```python
from build123d import *

# Parameters (mm, degrees)
ROW_SKETCH_W            = 16
ROW_SKETCH_H            = 6
ROW_ANGLE               = 59
HEEL_SKETCH_W           = 44
HEEL_SKETCH_H           = 6
HEEL_ANGLE              = 30
LUG_BLOCK_SKETCH_W      = 22
LUG_BLOCK_SKETCH_H      = 33
LUG_BLOCK_DEPTH         = 25
SLOT_SKETCH_W           = 32
SLOT_SKETCH_H           = 33
SLOT_DEPTH              = 20
PIN_HOLE_SKETCH_R       = 3.1
PIN_HOLE_DEPTH          = 30
TAB_SKETCH_W            = 23
TAB_SKETCH_H            = 26
TAB_DEPTH               = 5
SWITCH_HOLES_SKETCH_R   = 1.1
SWITCH_HOLES_DEPTH      = 30
SCREW_HOLE_1_SKETCH_R   = 2.25
SCREW_HOLE_1_DEPTH      = 200
SCREW_HOLE_1_SKETCH_2_R = 2.25
SCREW_HOLE_1_2_DEPTH    = 200


with BuildPart() as part:
    # Row Sketch → Row (revolve, symmetric)
    with BuildSketch(Plane.XY) as row_sk:
        with Locations((-896, 104.7)):
            Rectangle(ROW_SKETCH_W, ROW_SKETCH_H)
    revolve(axis=Axis((-3000, 0, 0), (1, 0, 0)), revolution_arc=ROW_ANGLE / 2)
    revolve(row_sk.sketch, axis=Axis((-3000, 0, 0), (-1, 0, 0)), revolution_arc=ROW_ANGLE / 2)

    # Heel Sketch → Heel (revolve, symmetric)
    with BuildSketch(Plane.XY) as heel_sk:
        with Locations((-866, 104.7)):
            Rectangle(HEEL_SKETCH_W, HEEL_SKETCH_H)
    revolve(axis=Axis((-3000, 0, 0), (1, 0, 0)), revolution_arc=HEEL_ANGLE / 2)
    revolve(heel_sk.sketch, axis=Axis((-3000, 0, 0), (-1, 0, 0)), revolution_arc=HEEL_ANGLE / 2)

    # Lug Block Sketch → Lug Block (add, symmetric)
    with BuildSketch(Plane.XY):
        with Locations((-856, 119.5)):
            Rectangle(LUG_BLOCK_SKETCH_W, LUG_BLOCK_SKETCH_H)
    extrude(amount=LUG_BLOCK_DEPTH, both=True)

    # Slot Sketch → Slot (cut, symmetric)
    with BuildSketch(Plane.XY):
        with Locations((-856, 124.5)):
            Rectangle(SLOT_SKETCH_W, SLOT_SKETCH_H)
    extrude(amount=SLOT_DEPTH, both=True, mode=Mode.SUBTRACT)

    # Pin Hole Sketch → Pin Hole (cut, symmetric)
    with BuildSketch(Plane.XY):
        with Locations((-856, 125)):
            Circle(PIN_HOLE_SKETCH_R)
    extrude(amount=PIN_HOLE_DEPTH, both=True, mode=Mode.SUBTRACT)

    # Tab Sketch → Tab (add)
    with BuildSketch(Plane.XY.offset(20)):
        with Locations((-856.5, 149)):
            Rectangle(TAB_SKETCH_W, TAB_SKETCH_H)
    extrude(amount=TAB_DEPTH)

    # Switch Holes Sketch → Switch Holes (cut, symmetric)
    with BuildSketch(Plane.XY):
        with Locations((-860.75, 155.6)):
            Circle(SWITCH_HOLES_SKETCH_R)
        with Locations((-851.25, 155.6)):
            Circle(SWITCH_HOLES_SKETCH_R)
    extrude(amount=SWITCH_HOLES_DEPTH, both=True, mode=Mode.SUBTRACT)

    # Screw Hole -1 Sketch → Screw Hole -1 (cut)
    with BuildSketch(Plane(origin=(0, 0, 0), x_dir=(-1, 0, 0), z_dir=(0, -0.9238795325112867, 0.38268343236508984))):
        with Locations(Location((896, 0, 0), (0, 0, 90))):
            Circle(SCREW_HOLE_1_SKETCH_R)
    extrude(amount=-SCREW_HOLE_1_DEPTH, mode=Mode.SUBTRACT)

    # Screw Hole 1 Sketch 2 → Screw Hole 1 2 (cut)
    with BuildSketch(Plane(origin=(0, 0, 0), x_dir=(-1, 0, 0), z_dir=(0, -0.9238795325112867, -0.3826834323650897))):
        with Locations(Location((896, 0, 0), (0, 0, 90))):
            Circle(SCREW_HOLE_1_SKETCH_2_R)
    extrude(amount=-SCREW_HOLE_1_2_DEPTH, mode=Mode.SUBTRACT)


solid = part.part
```
Part model, mm, in its own coordinate system. A direction names the side the tool comes from. Round coordinates to 2 decimals unless told otherwise and drop trailing zeros. Loops run counter-clockwise (first coordinate to the right, second up) from the corner with the lowest first, then second, coordinate; pieces in that order, holes last.
Item 1: Drop flat-ended pins along their axis: P1, Ø4, axis at x = -851.5, z = -22, coming from the +Y side; P2, Ø3, axis at x = -881, z = -16.5, coming from the +Y side; P3, Ø18.5, axis at x = -855.5, y = 136, coming from the -Z side; P4, Ø15.5, axis at y = 120, z = -5, coming from the -X side. Give the stop position or say it passes through.
Item 2: Cut at D-D, the plane z = -8.5. Give the cut face in (x, y), then the cut area to 3 significant figures.
Item 3: Cut at B-B, the plane y = 125. Give the cut face in (x, z), then the cut area to 3 significant figures.
Item 4: Mould opens along Z. For faces 1 (the face through (-896.1, 91.2, 51.6)), 2 (the face through (-904, 103, 0)), 3 (the face through (-898.196, 96.866, -39.595)) say: +Z half, -Z half, draft (parallel to the pull), parting line (faces both ways), or undercut.
Item 5: 3-axis set-ups, long thin cutter, end or side, ignore diameter. For faces 4 (the face through (-857, 134, 25)), 5 (the face through (-866.31, 101.17, -27.11)), 6 (the face through (-856, 121, -25)): which of +Z, -Z, +X, -X, +Y, -Y reach the whole face in a straight line?
Item 6: Cut at C-C, the plane x = -856. Give the cut face in (y, z), then the cut area to 3 significant figures.
Item 7: Drill centre lines: line 1 (X direction, y = 155.6, z = 21.95); line 2 (Z direction, x = -847.5, y = 118.5); line 3 (X direction, y = 155, z = 23). Where is each one in solid material? Low to high.
Item 8: Cut at A-A, the plane y = 112.5. Give the cut face in (x, z).
A:
1. P1: stops at y = 136
1. P2: stops at y = 106.65
1. P3: stops at z = -25
1. P4: passes through
2. outline: (-904, 101.34) - (-844, 101.34) - (-844, 107.36) - (-845, 107.36) - (-845, 108) - (-867, 108) - (-867, 107.36) - (-904, 107.36) - close
2. area: 375 mm2
3. outline: (-867, -25) - (-859.1, -25) - (-859.1, -20) - (-867, -20) - close; (-867, 20) - (-859.1, 20) - (-859.1, 25) - (-867, 25) - close; (-852.9, -25) - (-845, -25) - (-845, -20) - (-852.9, -20) - close; (-852.9, 20) - (-845, 20) - (-845, 25) - (-852.9, 25) - close
3. area: 158 mm2
4. face 1: +Z half
4. face 2: draft
4. face 3: undercut
5. face 4: +Z, +X, -X, +Y
5. face 5: -Z, +X, -Y
5. face 6: -Z, +X, -X, +Y
6. outline: (98.23, -26.32) - (104.03, -27.87) arc R107.7 ccw to (104.76, -25) - (121.9, -25) - (121.9, -20) - (108, -20) - (108, 20) - (121.9, 20) - (121.9, 25) - (104.76, 25) arc R107.7 ccw to (104.03, 27.87) - (98.23, 26.32) arc R101.7 cw to start; (128.1, -25) - (136, -25) - (136, -20) - (128.1, -20) - close; (128.1, 20) - (162, 20) - (162, 25) - (128.1, 25) - close
6. area: 741 mm2
7. line 1: x = -868 to -861.85, -859.65 to -852.35, -850.15 to -845
7. line 2: z = -25 to -20, 20 to 25
7. line 3: x = -868 to -861.67, -859.83 to -852.17, -850.33 to -845
8. outline: (-867, -25) - (-845, -25) - (-845, -20) - (-867, -20) - close; (-867, 20) - (-845, 20) - (-845, 25) - (-867, 25) - close
